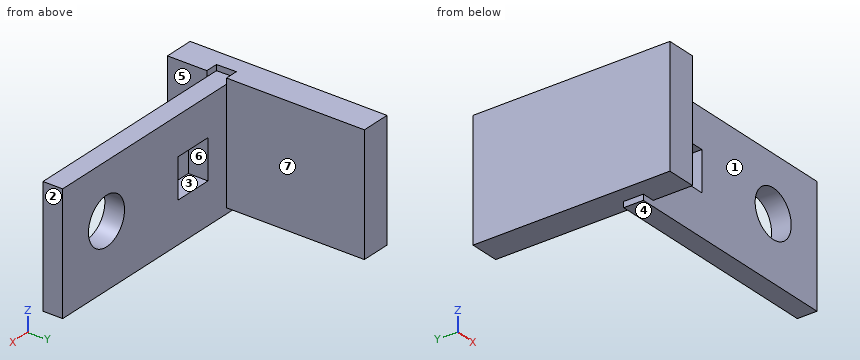
from build123d import *

# Parameters (mm, degrees)
F0_W     = 146.05
F0_H     = 76.2
F0_W_2   = 25.4
F0_H_2   = 25.4
F0_R     = 15.176992
F1_DEPTH = 12.7
F3_DEPTH = 76.2


with BuildPart() as f1:
    # F0 (on Front) → F1 (new body)
    with BuildSketch(Plane.XZ):
        with Locations((-16.311467, 34.471862)):
            Rectangle(F0_W, F0_H)
        with Locations((-52.800478, 35.423604)):
            Rectangle(F0_W_2, F0_H_2, mode=Mode.SUBTRACT)
        with Locations((19.859284, 37.236158)):
            Circle(F0_R, mode=Mode.SUBTRACT)
    extrude(amount=F1_DEPTH)

    # F2 (on Top) → F3 (join)
    with BuildSketch(Plane.XY):
        Polygon((-100.113213, -38.069502), (-81.063213, -38.069502), (-81.063213, -12.669502), (-89.156985, -12.669502), (-89.397579, 0), (-81.063213, 0), (-81.063213, 88.930498), (-100.113213, 88.930498), align=None)
    extrude(amount=F3_DEPTH)


solid = f1.part
Work out the finished part from the listing and answer in its coordinate system (mm). Face numbers are marked on the shaded views. A direction names the side the tool comes from. Coordinates: 2 decimals unless noted, no trailing zeros. Loops run counter-clockwise (first coordinate to the right, second up) from the corner with the lowest first, then second, coordinate; pieces in that order, holes last. Notation, with made-up numbers: (68.25, 80) -> (91.25, 80) arc R19 cw to (91.25, 99) -> close; hole circle Ø6 at (82.25, 71.5). An arc over 180 degrees is marked (long way). Write each question's results on one line, items separated by ' | '. Start each with the question number.
1) Find section C-C on y = -8.5. Determine the outline of the cut face in (x, z), then the cut area to 3 significant figures.
2) Find section A-A on z = 42. Determine the outline of the cut face in (x, y), then the cut area to 3 significant figures.
3) Consider line 1 along X through (y, z) = (5, 31); line 2 along Y through (x, z) = (-48, 70.5); line 3 along Z through (x, y) = (-84, -25). Determine where each line is inside the solid, lowest interval first.
4) Find section B-B on z = 50.5. Determine the outline of the cut face in (x, y).
5) For the marked faces 4, 5, 6 and 7, determine the directions among +Z, -Z, +X, -X, +Y, -Y from which every point of the face is accessible in a straight line to the end or side of a thin tool.
6) The mould has two halves that part along X. Classify the marked faces 1, 2 and 3: pulls with the +X half, pulls with the -X half, needs draft (parallel to the pull), parting line crosses it, or undercut.
7) Find section D-D on x = -71.5. Determine the outline of the cut face in (y, z), then the cut area to 3 significant figures.
8) Flat-ended cylindrical pins translate along their axes: P1, Ø7.5, axis at y = -24, z = 22, coming from the +X side; P2, Ø14, axis at x = 14, y = -8, coming from the +Z side; P3, Ø6, axis at x = 3.5, z = 19, coming from the +Y side. Find the tip coordinate at first contact, or state that the pin passes through.
Response values:
1) outline: (-100.11, 0) -> (-89.34, 0) -> (-89.34, -3.63) -> (56.71, -3.63) -> (56.71, 72.57) -> (-89.24, 72.57) -> (-89.24, 76.2) -> (-100.11, 76.2) -> close; hole (-65.5, 22.72) -> (-40.1, 22.72) -> (-40.1, 48.12) -> (-65.5, 48.12) -> close; hole circle Ø30.35 at (19.86, 37.24) | area: 10,600 mm^2
2) outline: (-100.11, -38.07) -> (-81.06, -38.07) -> (-81.06, -12.7) -> (-65.5, -12.7) -> (-65.5, 0) -> (-81.06, 0) -> (-81.06, 88.93) -> (-100.11, 88.93) -> close; (-40.1, -12.7) -> (5.45, -12.7) -> (5.45, 0) -> (-40.1, 0) -> close; (34.27, -12.7) -> (56.71, -12.7) -> (56.71, 0) -> (34.27, 0) -> close; hole (-89.4, 0) -> (-89.34, -3.22) -> (-89.34, 0) -> close | area: 3,480 mm^2
3) line 1: x = -100.11 to -81.06 | line 2: y = -12.7 to 0 | line 3: z = 0 to 76.2
4) outline: (-100.11, -38.07) -> (-81.06, -38.07) -> (-81.06, -12.7) -> (12.48, -12.7) -> (12.48, 0) -> (-81.06, 0) -> (-81.06, 88.93) -> (-100.11, 88.93) -> close; (27.24, -12.7) -> (56.71, -12.7) -> (56.71, 0) -> (27.24, 0) -> close; hole (-89.4, 0) -> (-89.34, -3.22) -> (-89.34, 0) -> close
5) face 4: -Z, +X, -X, +Y, -Y | face 5: +Z, -Z, +X, -Y | face 6: +Y, -Y | face 7: +Z, -Z, +X, +Y
6) face 1: needs draft | face 2: pulls with the +X half | face 3: undercut
7) outline: (-12.7, -3.63) -> (0, -3.63) -> (0, 72.57) -> (-12.7, 72.57) -> close | area: 968 mm^2
8) P1: stops at x = -81.06 | P2: stops at z = 72.57 | P3: stops at y = 0
